Source: CAD feature listing. Evaluate the final solid. Frame: model axes, mm. A direction names the side the tool comes from. Give positions to 0.01 mm unless a question says otherwise; leave off trailing zeros. Order: outer loops, then holes, each group sorted by start corner. A loop starts at its lowest first (then second) coordinate and runs counter-clockwise, first axis right, second up.
```python
from build123d import *

# Parameters (mm, degrees)
SKETCH1_R           = 13
SKETCH1_R_2         = 9.5
BOSS_EXTRUDE1_DEPTH = 15
SKETCH2_R           = 18
SKETCH2_R_2         = 9.5
BOSS_EXTRUDE2_DEPTH = 4
SKETCH3_R           = 9.5
SKETCH3_R_2         = 8.5
BOSS_EXTRUDE3_DEPTH = 2
SKETCH4_R           = 1.5
CUT_EXTRUDE1_DEPTH  = 32.764760349
SKETCH5_R           = 1
CUT_EXTRUDE2_DEPTH  = 8


with BuildPart() as part:
    # Sketch1 → Boss-Extrude1 (new body)
    with BuildSketch(Plane(origin=(0, 0, 0), x_dir=(0, 0, -1), z_dir=(1, 0, 0))):
        Circle(SKETCH1_R)
        Circle(SKETCH1_R_2, mode=Mode.SUBTRACT)
    extrude(amount=BOSS_EXTRUDE1_DEPTH)

    # Sketch2 → Boss-Extrude2 (add)
    with BuildSketch(Plane(origin=(15, 0, 0), x_dir=(0, 0, -1), z_dir=(1, 0, 0))):
        Circle(SKETCH2_R)
        Circle(SKETCH2_R_2, mode=Mode.SUBTRACT)
    extrude(amount=BOSS_EXTRUDE2_DEPTH)

    # Sketch3 → Boss-Extrude3 (add)
    with BuildSketch(Plane.ZY):
        Circle(SKETCH3_R)
        Circle(SKETCH3_R_2, mode=Mode.SUBTRACT)
    extrude(amount=-BOSS_EXTRUDE3_DEPTH)

    # Sketch4 → Cut-Extrude1 (cut, through all)
    with BuildSketch(Plane(origin=(19, 0, 0), x_dir=(0, 0, -1), z_dir=(1, 0, 0))):
        with Locations((0, 15)):
            Circle(SKETCH4_R)
        with Locations((15, 0)):
            Circle(SKETCH4_R)
        with Locations((0, -15)):
            Circle(SKETCH4_R)
        with Locations((-15, 0)):
            Circle(SKETCH4_R)
    extrude(amount=-CUT_EXTRUDE1_DEPTH, mode=Mode.SUBTRACT)

    # Sketch5 → Cut-Extrude2 (cut)
    with BuildSketch(Plane(origin=(19, 0, 0), x_dir=(0, 0, -1), z_dir=(1, 0, 0))):
        with Locations((7.919595949, 7.919595949)):
            Circle(SKETCH5_R)
        with Locations((7.919595949, -7.919595949)):
            Circle(SKETCH5_R)
        with Locations((-7.919595949, -7.919595949)):
            Circle(SKETCH5_R)
        with Locations((-7.919595949, 7.919595949)):
            Circle(SKETCH5_R)
    extrude(amount=-CUT_EXTRUDE2_DEPTH, mode=Mode.SUBTRACT)


solid = part.part
```
1) Section query D-D, the plane x = 2.5. Return the cut outline in (y, z), and give its area (3 significant figures).
Report:
outline: circle Ø26 at (0, 0); hole circle Ø19 at (0, 0)
area: 247 mm2
2) Reachability of faces 5 (the cylindrical face through (0.986, 7.167, 4.57)), 6 (the cylindrical face through (15.06, -8.53, 8.71)) from +Z, -Z, +X, -X, +Y, -Y: full face, straight path, thin tool, end or side. Return the list, or none.
Report:
face 5: +X, -X
face 6: +X
3) Section query A-A, the plane z = 0. Return the cut outline in (x, y), and give its area (3 significant figures).
Report:
outline: (0, -13) - (15, -13) - (15, -13.5) - (19, -13.5) - (19, -9.5) - (2, -9.5) - (2, -8.5) - (0, -8.5) - close; (0, 8.5) - (2, 8.5) - (2, 9.5) - (19, 9.5) - (19, 13.5) - (15, 13.5) - (15, 13) - (0, 13) - close; (15, -18) - (19, -18) - (19, -16.5) - (15, -16.5) - close; (15, 16.5) - (19, 16.5) - (19, 18) - (15, 18) - close
area: 153 mm2
4) Section query B-B, the plane z = 6. Return the cut outline in (x, y), and give its area (3 significant figures).
Report:
outline: (0, -11.53) - (15, -11.53) - (15, -16.97) - (19, -16.97) - (19, -7.37) - (2, -7.37) - (2, -6.02) - (0, -6.02) - close; (0, 6.02) - (2, 6.02) - (2, 7.37) - (19, 7.37) - (19, 16.97) - (15, 16.97) - (15, 11.53) - (0, 11.53) - close
area: 207 mm2
5) Material intervals for L1, parallel to Y at x = 17, z = 0; L2, parallel to Y at x = 8.75, z = 0; L3, parallel to Y at x = 16.75, z = -8, sorted ascending.
Report:
L1: y = -18 to -16.5, -13.5 to -9.5, 9.5 to 13.5, 16.5 to 18
L2: y = -13 to -9.5, 9.5 to 13
L3: y = -16.12 to -8.92, -6.92 to -5.12, 5.12 to 6.92, 8.92 to 16.12
6) Section query C-C, the plane y = -15. Return the cut outline in (x, z).
Report:
outline: (15, -9.95) - (19, -9.95) - (19, -1.5) - (15, -1.5) - close; (15, 1.5) - (19, 1.5) - (19, 9.95) - (15, 9.95) - close
7) Pin query (flat end, axial travel): pin 1 (2 mm diameter, centred on x = 6, z = -4, fed in from -Y); pin 2 (10 mm diameter, centred on x = 16, z = 3.5, fed in from +Y); pin 3 (1 mm diameter, centred on y = -8, z = 8, fed in from +X); pin 4 (15.5 mm diameter, centred on y = 0, z = 0, fed in from +X). Return the tip coordinate at first contact, or that it passes through.
Report:
pin 1: stops at y = -12.65
pin 2: stops at y = 18
pin 3: stops at x = 11
pin 4: passes through
8) Draft query along Y for faces 1 (the cylindrical face through (7.395, -7.91, 10.316)), 2 (the flat face through (15, -11, -8)), 3 (the cylindrical face through (15.056, -8.303, -8.843)), 4 (the cylindrical face through (17.03, 0.07, -13.5)). Return one class per face: +Y half, -Y half, draft (parallel to the pull), parting line (faces both ways), or undercut.
Report:
face 1: parting line
face 2: draft
face 3: undercut
face 4: undercut
